```python
from build123d import *

# Parameters (mm, degrees)
HOLE_WIZARD_M82_D = 6.8
CHAMFER_1_SIZE    = 1


with BuildPart() as part:
    # Эскиз1 → Повернуть1 (revolve)
    with BuildSketch(Plane.XY, mode=Mode.PRIVATE) as revolve_1_sk:
        Polygon((0, 3), (0, 9.25), (18, 9.25), (18, 8), (30, 8), (30, 3), align=None)
    revolve(revolve_1_sk.sketch.rotate(Axis((0, 0, 0), (1, 0, 0)), 90), axis=Axis((0, 0, 0), (1, 0, 0)))

    # Отверстие обработанное метчиком M82 (through all)
    with Locations(Plane.ZY):
        with Locations((0, 0)):
            Hole(HOLE_WIZARD_M82_D / 2)

    # Фаска1
    chamfer_1_edges = [part.edges().sort_by_distance(p)[0] for p in [
        (30, 0, -8),
        (0, 0, -9.25),
    ]]
    chamfer(chamfer_1_edges, length=CHAMFER_1_SIZE)


solid = part.part
```
The listing builds one solid part. Answer for the finished solid, in the listing's coordinates (mm). A direction names the side the tool comes from. Round coordinates to 2 decimals unless told otherwise and drop trailing zeros. Loops run counter-clockwise (first coordinate to the right, second up) from the corner with the lowest first, then second, coordinate; pieces in that order, holes last. Notation, with made-up numbers: (-39, 67.5) - (-6, 67.5) arc R29 cw to (-6, 106.5) - close; hole circle Ø2 at (49.5, 76). An arc over 180 degrees is marked (long way). Use one line per item in the form item = value. Start each with the question number.
1. The part is cut by section C-C on x = 5.5. Determine the outline of the cut face in (y, z).
2. The part is cut by section A-A on z = 0. Determine the outline of the cut face in (x, y).
3. For a pull along Z with two mould halves and no side action, classify faces 3 (the face through (0, 0, -4)), 4 (the face through (23.58, 7.81, -1.73)), 5 (the face through (15.21, -3.32, 0.74)) as pulls with the +Z half, pulls with the -Z half, needs draft (parallel to the pull), parting line crosses it, or undercut.
4. The part is cut by section D-D on x = 21. Determine the outline of the cut face in (y, z).
5. Given pin 1 Ø1.5 at (x, z) = (21, 6) entering from -Y; pin 2 Ø5 at (x, z) = (19.5, -4) entering from -Y; pin 3 Ø2 at (x, y) = (8, -2.5) entering from +Z, each flat-ended and moving along its own axis, determine where each tip first touches the part or whether it passes through.
6. A tool of negligible diameter and unlimited length cuts with its end or side. For faces 1 (the face through (18, -8, -3)), 2 (the face through (30, -2, 3)), from which of +Z, -Z, +X, -X, +Y, -Y can it reach the whole face along a straight path? Write none if from no direction.
7. Consider line 1 (Y direction, x = 21, z = 0); line 2 (Y direction, x = 15, z = 0); line 3 (Z direction, x = 4.5, y = 2.5). Determine where each line is inside the solid, lowest interval first. Write a range as [from, to].
Geometry check:
q1.outline = circle Ø18.5 at (0, 0); hole circle Ø6.8 at (0, 0)
q2.outline = (0, -8.25) - (1, -9.25) - (18, -9.25) - (18, -8) - (29, -8) - (30, -7) - (30, -3.4) - (0, -3.4) - close; (0, 3.4) - (30, 3.4) - (30, 7) - (29, 8) - (18, 8) - (18, 9.25) - (1, 9.25) - (0, 8.25) - close
q3.face_3 = needs draft
q3.face_4 = parting line crosses it
q3.face_5 = undercut
q4.outline = circle Ø16 at (0, 0); hole circle Ø6.8 at (0, 0)
q5.pin_1 = -6.04
q5.pin_2 = -9.03
q5.pin_3 = 9.13
q6.face_1 = +X
q6.face_2 = +Z, -Z, +X, +Y, -Y
q7.line_1 = [-8, -3.4], [3.4, 8]
q7.line_2 = [-9.25, -3.4], [3.4, 9.25]
q7.line_3 = [-8.91, -2.3], [2.3, 8.91]
